```python
from build123d import *

# Parameters (mm, degrees)
F1_DEPTH = 18
F3_DEPTH = 2
F6_D     = 8.5
F7_D     = 6.8
F7_DEPTH = 10
F7_TIP   = 2.0429261047


with BuildPart() as f1:
    # F0 (on Top) → F1 (new body)
    with BuildSketch(Plane.XY):
        with BuildLine():
            Line((-8.5, 9.1651513899), (-8.5, -9.1651513899))
            ThreePointArc((-8.5, -9.1651513899), (12.5, 0), (-8.5, 9.1651513899))
        make_face()
    extrude(amount=F1_DEPTH)

    # F2 (on face) → F3 (join)
    with BuildSketch(Plane.XY.offset(18)):
        with BuildLine():
            Line((-4.5, -7.5), (4.5, -7.5))
            ThreePointArc((4.5, -7.5), (6.6213203436, -6.6213203436), (7.5, -4.5))
            Line((7.5, -4.5), (7.5, 4.5))
            ThreePointArc((7.5, 4.5), (6.6213203436, 6.6213203436), (4.5, 7.5))
            Line((4.5, 7.5), (-4.5, 7.5))
            ThreePointArc((-4.5, 7.5), (-6.6213203436, 6.6213203436), (-7.5, 4.5))
            Line((-7.5, 4.5), (-7.5, -4.5))
            ThreePointArc((-7.5, -4.5), (-6.6213203436, -6.6213203436), (-4.5, -7.5))
        make_face()
    extrude(amount=F3_DEPTH)

    # F6 (through all)
    with Locations(Plane(origin=(-8.5, 0, 0), x_dir=(0, -1, 0), z_dir=(-1, 0, 0))):
        with Locations((0, 9)):
            Hole(F6_D / 2)

    # F7
    with Locations(Plane.XY.offset(20)):
        with Locations((0, 0)):
            Hole(F7_D / 2, depth=F7_DEPTH)
            with Locations((0, 0, -(F7_DEPTH + F7_TIP / 2))):  # 118° drill point
                Cone(0, F7_D / 2, F7_TIP, mode=Mode.SUBTRACT)


solid = f1.part
```
Source: CAD feature listing. Evaluate the final solid. Frame: model axes, mm. A direction names the side the tool comes from. Coordinates: 2 decimals unless noted, no trailing zeros. Loops run counter-clockwise (first coordinate to the right, second up) from the corner with the lowest first, then second, coordinate; pieces in that order, holes last. Notation, with made-up numbers: M -1.5,20 L 24.5,20 A20 ccw 24.5,52 Z; hole C 43.5,83 d1. An arc over 180 degrees is marked long. Use a Markdown table: item, result. Add a question column.
Q1. Section query A-A, the plane y = 0. Return loops of the section in (x, z).
Q2. Section query C-C, the plane x = 8.5. Return loops of the section in (y, z), and give its area (3 significant figures).
Q3. First-contact query: pin 1 (0.6 mm diameter, centred on y = -1, z = 18.5, fed in from -X); pin 2 (0.6 mm diameter, centred on y = -1.5, z = 19, fed in from +X); pin 3 (2 mm diameter, centred on x = 6, z = 4, fed in from +Y). Flat tips, straight axial feed; report the tip coordinate or a pass-through.
Q4. Draft query along X for faces 1 (the cylindrical face through (3.4, 0.1, 16.7)), 2 (the flat face through (-8.5, -2, 13)), 3 (the cylindrical face through (10.67, -6.51, 8.87)), 4 (the flat face through (9, 0, 18)). Return one class per face: pulls with the +X half, pulls with the -X half, needs draft (parallel to the pull), parting line crosses it, or undercut.
Q5. Material intervals for L1, parallel to Y at x = 0, z = 16; L2, parallel to Z at x = 6.75, y = -0.25; L3, parallel to X at y = 0, z = 15.5, sorted ascending.
Q6. Section query D-D, the plane z = 9. Return loops of the section in (x, y), and give its area (3 significant figures).
Q7. Section query B-B, the plane x = 0. Return loops of the section in (y, z).
Q8. Access query for faces 5 (the cylindrical face through (6.64, 6.6, 18.99)), 6 (the cylindrical face through (-6.64, -6.6, 18.99)), 7 (the cylindrical face through (-6.6, 6.64, 18.99)). Directions: +Z, -Z, +X, -X, +Y, -Y. A direction counts if a zero-diameter tool reaches every point of the face in a straight line with its end or side. Return the directions, or none.
Result:
| question | item | result |
|---|---|---|
| 1 | outline | M -8.5,0 L 12.5,0 L 12.5,4.75 L -8.5,4.75 Z; M -8.5,13.25 L -3.4,13.25 L -3.4,20 L -7.5,20 L -7.5,18 L -8.5,18 Z; M 3.4,13.25 L 12.5,13.25 L 12.5,18 L 7.5,18 L 7.5,20 L 3.4,20 Z |
| 2 | outline | M -9.17,0 L 9.17,0 L 9.17,18 L -9.17,18 Z; hole C 0,9 d8.5 |
| 2 | area | 273 mm2 |
| 3 | pin 1 | stops at x = -7.5 |
| 3 | pin 2 | stops at x = 7.5 |
| 3 | pin 3 | stops at y = 11.46 |
| 4 | face 1 | undercut |
| 4 | face 2 | pulls with the -X half |
| 4 | face 3 | parting line crosses it |
| 4 | face 4 | needs draft |
| 5 | L1 | y = -12.5 to -3.4, 3.4 to 12.5 |
| 5 | L2 | z = 0 to 4.76, 13.24 to 20 |
| 5 | L3 | x = -8.5 to -3.4, 3.4 to 12.5 |
| 6 | outline | M -8.5,-9.17 A12.5 ccw 11.76,-4.25 L -8.5,-4.25 Z; M -8.5,4.25 L 11.76,4.25 A12.5 ccw -8.5,9.17 Z |
| 6 | area | 264 mm2 |
| 7 | outline | M -12.5,0 L 12.5,0 L 12.5,18 L 7.5,18 L 7.5,20 L 3.4,20 L 3.4,11.55 A4.25 cw long -3.4,11.55 L -3.4,20 L -7.5,20 L -7.5,18 L -12.5,18 Z |
| 8 | face 5 | +Z, +X, +Y |
| 8 | face 6 | +Z, -X, -Y |
| 8 | face 7 | +Z, -X, +Y |
